Part model, mm, in its own coordinate system. Face numbers are marked on the shaded views. A direction names the side the tool comes from. Give positions to 0.01 mm unless a question says otherwise; leave off trailing zeros. Write each loop counter-clockwise with the first axis right and the second up, starting at its lowest first coordinate (ties: lowest second). Pieces come first, ordered by that corner, then holes. Notation, with made-up numbers: M -34,86.25 L 11,86.25 A10 cw 11,99.25 Z; hole C 32,39.5 d7. An arc over 180 degrees is marked long. Use a Markdown table: item, result. Add a question column.
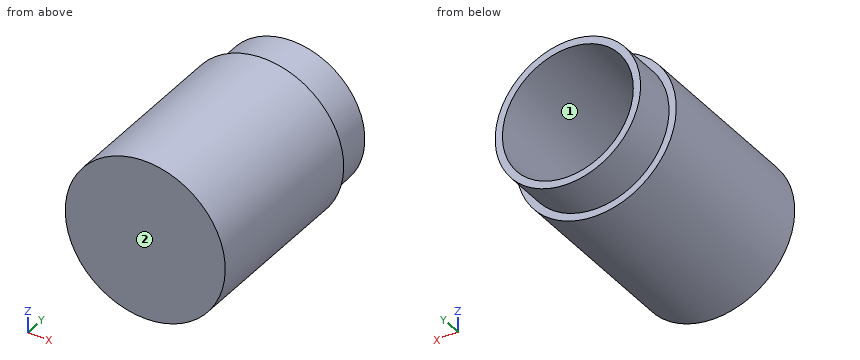
from build123d import *

# Parameters (mm, degrees)
SKETCH1_R           = 45
BOSS_EXTRUDE2_DEPTH = 150
SHELL1_T            = 5
SKETCH2_R           = 55
SKETCH2_R_2         = 50
BOSS_EXTRUDE3_DEPTH = 125


with BuildPart() as part:
    # Sketch1 → Boss-Extrude2 (new body)
    with BuildSketch(Plane(origin=(0, 0, 0), x_dir=(1, 0, 0), z_dir=(0, 1, 0))):
        with Locations(Location((0, 0, 0), (0, 0, 270))):
            Circle(SKETCH1_R)
    extrude(amount=BOSS_EXTRUDE2_DEPTH)

    # Shell1
    shell1_openings = [part.faces().sort_by_distance(p)[0] for p in [
        (0, 150, 0),
    ]]
    offset(amount=SHELL1_T, openings=shell1_openings, kind=Kind.INTERSECTION)

    # Sketch2 → Boss-Extrude3 (add)
    with BuildSketch(Plane(origin=(0, -5, 0), x_dir=(-1, 0, 0), z_dir=(0, -1, 0))):
        with Locations(Location((0, 0, 0), (0, 0, 90))):
            Circle(SKETCH2_R)
        with Locations(Location((0, 0, 0), (0, 0, 90))):
            Circle(SKETCH2_R_2, mode=Mode.SUBTRACT)
    extrude(amount=-BOSS_EXTRUDE3_DEPTH)


solid = part.part
1. Cut at C-C (y = 79). Write the cut outline in (x, z).
2. Tool access for the marked faces 1 and 2: list every direction of +Z, -Z, +X, -X, +Y, -Y with a clear straight run to the whole face (end or side of a thin tool).
3. Cut at A-A (x = 0). Write the cut outline in (y, z).
4. Drill centre lines: probe 1 along X at (y, z) = (109, 0); probe 2 along Y at (x, z) = (31, -15); probe 3 along Z at (x, y) = (-11, 2.5). Where is each one in solid material? Low to high. Write a range as [from, to].
5. Cut at B-B (z = 0). Write the cut outline in (x, y), then the cut area to 3 significant figures.
6. Cut at D-D (z = 47.5). Write the cut outline in (x, y), then the cut area to 3 significant figures.
7. Flat gauge pins, fed straight in: pin 1 (10 mm diameter, centred on x = 12.5, y = 82.5, fed in from +Z); pin 2 (4 mm diameter, centred on x = 27, y = 78.5, fed in from +Z); pin 3 (1.5 mm diameter, centred on x = 41, y = 28.5, fed in from +Z). Where does each tip first touch, or does it go through?
A:
| question | item | result |
|---|---|---|
| 1 | outline | C 0,0 d110; hole C 0,0 d90 |
| 2 | face 1 | +Y |
| 2 | face 2 | +Z, -Z, +X, -X, -Y |
| 3 | outline | M -5,-55 L 120,-55 L 120,-50 L 150,-50 L 150,-45 L 0,-45 L 0,45 L 150,45 L 150,50 L 120,50 L 120,55 L -5,55 Z |
| 4 | probe 1 | x = [-55, -45], [45, 55] |
| 4 | probe 2 | y = [-5, 0] |
| 4 | probe 3 | z = [-53.89, -43.63], [43.63, 53.89] |
| 5 | outline | M -55,-5 L 55,-5 L 55,120 L 50,120 L 50,150 L 45,150 L 45,0 L -45,0 L -45,150 L -50,150 L -50,120 L -55,120 Z |
| 5 | area | 3,250 mm² |
| 6 | outline | M -27.73,-5 L 27.73,-5 L 27.73,120 L 15.61,120 L 15.61,150 L -15.61,150 L -15.61,120 L -27.73,120 Z |
| 6 | area | 7,870 mm² |
| 7 | pin 1 | stops at z = 54.49 |
| 7 | pin 2 | stops at z = 48.99 |
| 7 | pin 3 | stops at z = 37.48 |
